Could you check a few things on this model? Use its own coordinates, in mm. Face numbers are marked on the shaded views. Give positions to 0.01 mm unless a question says otherwise; leave off trailing zeros. Order: outer loops, then holes, each group sorted by start corner. A loop starts at its lowest first (then second) coordinate and runs counter-clockwise, first axis right, second up. Notation, with made-up numbers: (17.5, 17.25) -> (57.5, 17.25) arc R8 cw to (57.5, 28.25) -> close; hole circle Ø9 at (59.25, 89.5). An arc over 180 degrees is marked (long way). Use one line per item in the form item = value. Start each with the question number.
from build123d import *

# Parameters (mm, degrees)
BOSS_EXTRUDE1_DEPTH = 1
SKETCH2_R           = 2.775
BOSS_EXTRUDE2_DEPTH = 3
BOSS_EXTRUDE3_DEPTH = 2


with BuildPart() as part:
    # Sketch1 → Boss-Extrude1 (new body)
    with BuildSketch(Plane.XY):
        Polygon((-1.71944816, -3.077706513), (-1.71944816, -1.63433084), (-2.96944816, -0.912643004), (-4.21944816, -1.63433084), (-4.21944816, -3.077706513), (-2.96944816, -3.79939435), align=None)
    extrude(amount=BOSS_EXTRUDE1_DEPTH)



with BuildPart() as body_2:
    # Sketch2 → Boss-Extrude2 (new body)
    with BuildSketch(Plane.XY.offset(1)):
        Polygon((-2.96944816, -6.856018677), (0.927666157, -4.606018677), (0.927666157, -0.106018677), (-2.96944816, 2.143981323), (-6.866562477, -0.106018677), (-6.866562477, -4.606018677), align=None)
        with Locations((-2.96944816, -2.356018677)):
            Circle(SKETCH2_R, mode=Mode.SUBTRACT)
    extrude(amount=-BOSS_EXTRUDE2_DEPTH)


with BuildPart() as part_1:
    add(part.part)

    add(body_2.part)  # Boss-Extrude3 merges body 2
    # Sketch3 → Boss-Extrude3 (add)
    with BuildSketch(Plane.XY.offset(1)):
        Polygon((-2.96944816, -6.856018677), (0.927666157, -4.606018677), (0.927666157, -0.106018677), (-2.96944816, 2.143981323), (-6.866562477, -0.106018677), (-6.866562477, -4.606018677), align=None)
    extrude(amount=BOSS_EXTRUDE3_DEPTH)


solid = part_1.part
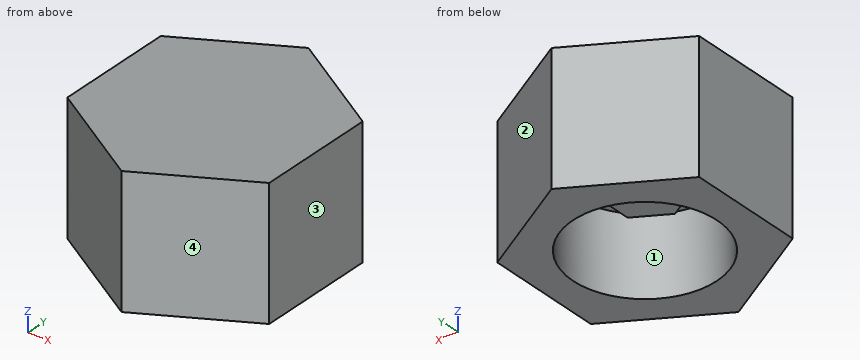
(1) We'd pull the mould along Y, two halves only. Please class the marked faces 1, 2, 3 and 4: pulls with the +Y half, pulls with the -Y half, needs draft (parallel to the pull), parting line crosses it, or undercut.
(2) I'm going to push a flat-ended pin straight in: pin 1 Ø0.8 at (x, y) = (-3.5, -2.5) entering from -Z. Where does the tip first touch, or does it pass through?
(3) Imagine slicing it at C-C (x = -2). Write out the boundary of the cut face in (y, z), plus the area to 3 significant figures.
(4) Imagine slicing it at A-A (z = 0.5). Write out the boundary of the cut face in (x, y) (3 decimals).
(5) Please list where these lines run through material, in increasing order: probe 1 along Z at (x, y) = (-0.75, -2.5); probe 2 along X at (y, z) = (-2, 0.9); probe 3 along Y at (x, z) = (-2.5, -0.5).
(6) Imagine slicing it at B-B (z = -1.45). Write out the boundary of the cut face in (x, y) (3 decimals).
(7) Imagine slicing it at D-D (y = -4.5). Write out the boundary of the cut face in (x, z), plus the area to 3 significant figures.
Calculated:
q1.face_1 = undercut
q1.face_2 = pulls with the +Y half
q1.face_3 = needs draft
q1.face_4 = pulls with the -Y half
q2.pin_1 = 0
q3.outline = (-6.3, -2) -> (-4.96, -2) -> (-4.96, 1) -> (-3.24, 1) -> (-3.24, 0) -> (-1.47, 0) -> (-1.47, 1) -> (0.24, 1) -> (0.24, -2) -> (1.58, -2) -> (1.58, 3) -> (-6.3, 3) -> close
q3.area = 25.6 mm2
q4.outline = (-6.867, -4.606) -> (-2.969, -6.856) -> (0.928, -4.606) -> (0.928, -0.106) -> (-2.969, 2.144) -> (-6.867, -0.106) -> close; (-4.219, -3.078) -> (-2.969, -3.799) -> (-1.719, -3.078) -> (-1.719, -1.634) -> (-2.969, -0.913) -> (-4.219, -1.634) -> close; hole circle Ø5.55 at (-2.969, -2.356)
q5.probe_1 = 1 to 3
q5.probe_2 = -6.87 to -5.72, -4.22 to -1.72, -0.22 to 0.93
q5.probe_3 = -6.58 to -5.09, 0.38 to 1.87
q6.outline = (-6.867, -4.606) -> (-2.969, -6.856) -> (0.928, -4.606) -> (0.928, -0.106) -> (-2.969, 2.144) -> (-6.867, -0.106) -> close; hole circle Ø5.55 at (-2.969, -2.356)
q7.outline = (-6.87, -2) -> (-4.73, -2) -> (-4.73, 1) -> (-1.21, 1) -> (-1.21, -2) -> (0.93, -2) -> (0.93, 3) -> (-6.87, 3) -> close
q7.area = 28.4 mm2
